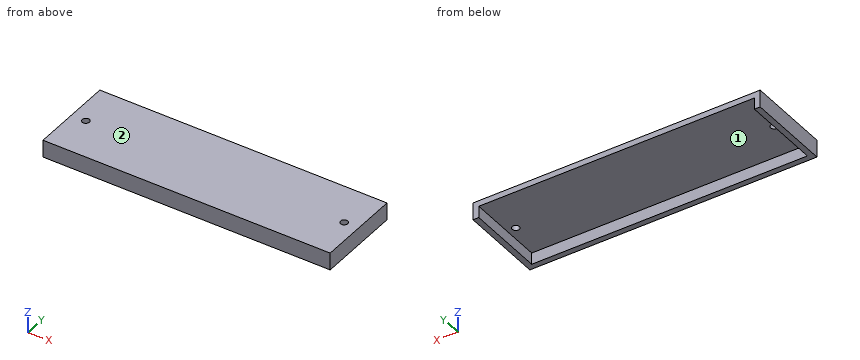
Autodesk Inventor part; units mm, degrees
ref_plane "Pracovní rovina11" through (0, 0, 164) normal (0, 0, 1) x (1, 0, 0)
ref_plane "YZ Plane" through (0, 0, 0) normal (1, 0, 0) x (0, 1, 0)
ref_plane "XZ Plane" through (0, 0, 0) normal (0, 1, 0) x (-1, 0, 0)
ref_plane "Pracovní rovina11" through (0, 0, 164) normal (0, 0, 1) x (1, 0, 0)
sketch "Náčrt11" plane through (0, 0, 164) normal (0, 0, 1) x (1, 0, 0)
  line L0 (-0.5, -50.5) -> (190.5, -50.5)
  line L1 (190.5, -50.5) -> (190.5, 0.5)
  line L2 (190.5, 0.5) -> (-0.5, 0.5)
  line L3 (-0.5, 0.5) -> (-0.5, -50.5)
  line L4 (0, 0) -> (0, -50)
  line L5 (190, -50) -> (190, 0)
  line L6 (190, 0) -> (0, 0)
  line L7 (182, -50) -> (58, -50)
  line L8 (-4.5, 4.5) -> (194.5, 4.5)
  line L9 (194.5, 4.5) -> (194.5, -54.5)
  line L10 (194.5, -54.5) -> (-4.5, -54.5)
  line L11 (-4.5, -54.5) -> (-4.5, 4.5)
  dimension "d43" = 0.5
  dimension "d44" = 0.5
  dimension "d45" = 0.5
  dimension "d46" = 0.5
  dimension "d47" = 4
extrude "Vysunutí11" add sketch "Náčrt11" against normal blind 8
sketch "Náčrt12" plane through (0, 0, 164) normal (0, 0, 1) x (1, 0, 0)
  line L0 (-4.5, 4.5) -> (-4.5, -54.5)
  line L1 (194.5, 4.5) -> (-4.5, 4.5)
  line L2 (194.5, -54.5) -> (194.5, 4.5)
  line L3 (-4.5, -54.5) -> (194.5, -54.5)
  point P0 (0, 0)
extrude "Vysunutí12" add sketch "Náčrt12" along normal blind 4
sketch "Náčrt13" plane through (0, 0, 168) normal (0, 0, 1) x (1, 0, 0)
  circle A0 centre (5.5, -25) radius 2.5
  circle A1 centre (184.5, -25) radius 2.5
  line L0 (-4.5, -54.5) -> (194.5, -54.5)
  line L1 (194.5, 4.5) -> (-4.5, 4.5)
  line L2 (-4.5, 4.5) -> (-4.5, -54.5)
  line L3 (194.5, -54.5) -> (194.5, 4.5)
  point P0 (0, 0)
  dimension "d52" = 5
  dimension "d53" = 5
  dimension "d54" = 59
  dimension "d55" = 29.5
  dimension "d56" = 29.5
  dimension "d57" = 10
  dimension "d58" = 10
extrude "Vysunutí13" cut sketch "Náčrt13" against normal through all contours A0 | A1
sketch "Náčrt14" plane through (-4.5, 4.5, 156) normal (0, 1, 0) x (1, 0, 0)
  line L0 (4, -8) -> (4, 0)
  line L1 (195, -8) -> (195, 0)
  line L2 (4, -8) -> (195, -8)
  line L3 (0, 0) -> (199, 0)
  point P0 (4.5, 156)
extrude "Vysunutí14" cut sketch "Náčrt14" against normal up to surface (4 mm away)
properties part number "krab1"
The model under review builds one solid part; all positions refer to its coordinate system, in mm. Face numbers are marked on the shaded views. Coordinates: 2 decimals unless noted, no trailing zeros. Loops run counter-clockwise (first coordinate to the right, second up) from the corner with the lowest first, then second, coordinate; pieces in that order, holes last.
(1) Draft analysis for pull direction X (two halves, no side actions). For the marked faces 1 and 2, state which applies: +X half, -X half, draft (parallel to the pull), parting line (faces both ways), or undercut.
Determined:
face 1: undercut
face 2: draft
(2) Consider section D-D, the plane y = -16. Give the boundary of the cut face in (x, z), plus the area to 3 significant figures.
Determined:
outline: (-4.5, 156) - (-0.5, 156) - (-0.5, 164) - (190.5, 164) - (190.5, 156) - (194.5, 156) - (194.5, 168) - (-4.5, 168) - close
area: 860 mm2
(3) Consider section B-B, the plane x = 184.5. Give the boundary of the cut face in (y, z), plus the area to 3 significant figures.
Determined:
outline: (-54.5, 156) - (-50.5, 156) - (-50.5, 164) - (-27.5, 164) - (-27.5, 168) - (-54.5, 168) - close; (-22.5, 164) - (4.5, 164) - (4.5, 168) - (-22.5, 168) - close
area: 248 mm2
(4) Wall thickness on L1, parallel to X at y = -48.5, z = 162.75; L2, parallel to Y at x = 5.5, z = 165.25; L3, parallel to Z at x = 180.5, y = -48: over which ranges is each line inside the solid? List them lowest first.
Determined:
L1: x = -4.5 to -0.5, 190.5 to 194.5
L2: y = -54.5 to -27.5, -22.5 to 4.5
L3: z = 164 to 168
(5) Consider section C-C, the plane z = 158.25. Give the boundary of the cut face in (x, y).
Determined:
outline: (-4.5, -54.5) - (194.5, -54.5) - (194.5, 4.5) - (190.5, 4.5) - (190.5, -50.5) - (-0.5, -50.5) - (-0.5, 4.5) - (-4.5, 4.5) - close
(6) Insertion check: P1, Ø16.5, axis at x = 58, y = -35, coming from the -Z side; P2, Ø2.5, axis at x = 109.5, z = 161, coming from the +Y side. Each pin has a flat end and moves straight along its axis. Give the tip position at first contact, or say it passes through.
Determined:
P1: stops at z = 164
P2: stops at y = -50.5
(7) Consider section A-A, the plane y = -25. Give the boundary of the cut face in (x, z).
Determined:
outline: (-4.5, 156) - (-0.5, 156) - (-0.5, 164) - (3, 164) - (3, 168) - (-4.5, 168) - close; (8, 164) - (182, 164) - (182, 168) - (8, 168) - close; (187, 164) - (190.5, 164) - (190.5, 156) - (194.5, 156) - (194.5, 168) - (187, 168) - close
